```python
from build123d import *

# Parameters (mm, degrees)
F0_W     = 26
F0_H     = 15
F0_R     = 1.7
F1_DEPTH = 1.5
F2_W     = 5
F2_H     = 5
F2_R     = 1.7
F2_H_2   = 3
F3_DEPTH = 2
F4_R     = 1


with BuildPart() as f1:
    # F0 (on Top) → F1 (new body)
    with BuildSketch(Plane.XY):
        with Locations((-13, -7.5)):
            Rectangle(F0_W, F0_H)
        with Locations((-22.5, -11.9)):
            Circle(F0_R, mode=Mode.SUBTRACT)
        with Locations((-3.5, -11.9)):
            Circle(F0_R, mode=Mode.SUBTRACT)
    extrude(amount=F1_DEPTH)

    # F2 (on face) → F3 (join)
    with BuildSketch(Plane.XY.offset(1.5)):
        with Locations((-22.5, -11.9)):
            Rectangle(F2_W, F2_H)
        with Locations((-22.5, -11.9)):
            Circle(F2_R, mode=Mode.SUBTRACT)
        with Locations((-3.5, -11.9)):
            Rectangle(F2_W, F2_H)
        with Locations((-3.5, -11.9)):
            Circle(F2_R, mode=Mode.SUBTRACT)
        with Locations((-22.5, -1.5)):
            Rectangle(F2_W, F2_H_2)
        with Locations((-3.5, -1.5)):
            Rectangle(F2_W, F2_H_2)
    extrude(amount=F3_DEPTH)

    # F4
    f4_edges = [f1.edges().sort_by_distance(p)[0] for p in [
        (-26, 0, 0.75),
        (-26, -15, 0.75),
        (0, -15, 0.75),
        (0, 0, 0.75),
        (-1, -3, 2.5),
        (-6, -3, 2.5),
        (-20, -3, 2.5),
        (-25, -3, 2.5),
        (-25, -14.4, 2.5),
        (-25, -9.4, 2.5),
        (-20, -9.4, 2.5),
        (-20, -14.4, 2.5),
        (-6, -14.4, 2.5),
        (-1, -14.4, 2.5),
        (-1, -9.4, 2.5),
        (-6, -9.4, 2.5),
    ]]
    fillet(f4_edges, radius=F4_R)


solid = f1.part
```
Geometry: final body of the model. Coordinates: model frame, mm. A direction names the side the tool comes from. Round coordinates to 2 decimals unless told otherwise and drop trailing zeros. Order: outer loops, then holes, each group sorted by start corner. A loop starts at its lowest first (then second) coordinate and runs counter-clockwise, first axis right, second up. Notation, with made-up numbers: M 6,-25 L 28,-25 A29 ccw 28,-2 Z; hole C 0,-19.75 d8. An arc over 180 degrees is marked long. One line per item, written item: value.
(1) Cut plane A-A (z = 2.4). Give the number of separate pieces and of enclosed holes in the cut face, and give its area (3 significant figures).
Result sheet:
separate pieces: 4
enclosed holes: 2
area: 59.3 mm2
(2) Reachability of faces 5 (the cylindrical face through (-24.715, -9.701, 2.514)), 6 (the flat face through (-4, -9.4, 2)), 7 (the flat face through (-6, -12, 2)), 8 (the cylindrical face through (-1.285, -14.099, 2.514)), 9 (the flat face through (-13, -7, 1.5)) from +Z, -Z, +X, -X, +Y, -Y: full face, straight path, thin tool, end or side. Return the list, or none.
Result sheet:
face 5: +Z, -X
face 6: +Z, +X, -X
face 7: +Z, +Y, -Y
face 8: +Z, +X, -Y
face 9: +Z
(3) Pin query (flat end, axial travel): P1, Ø2, axis at y = -2.5, z = 3, coming from the +X side; P2, Ø1.6, axis at y = -11.5, z = 2.5, coming from the -X side; P3, Ø1.6, axis at x = -3.5, z = 3, coming from the -Y side. Return the tip coordinate at first contact, or that it passes through.
Result sheet:
P1: x = -1
P2: x = -25
P3: y = -14.4
(4) Cut plane B-B (x = -22.5). Return the cut outline in (y, z).
Result sheet:
outline: M -15,0 L -13.6,0 L -13.6,3.5 L -14.4,3.5 L -14.4,1.5 L -15,1.5 Z; M -10.2,0 L 0,0 L 0,3.5 L -3,3.5 L -3,1.5 L -9.4,1.5 L -9.4,3.5 L -10.2,3.5 Z
(5) Line query: probe 1 along Y at (x, z) = (-22.5, 2.8); probe 2 along X at (y, z) = (-11.75, 1.65); probe 3 along Y at (x, z) = (-3.5, 1.05). Output: solid intervals per line, ascending. Write a range as [from, to].
Result sheet:
probe 1: [-14.4, -13.6], [-10.2, -9.4], [-3, 0]
probe 2: [-25, -24.19], [-20.81, -20], [-6, -5.19], [-1.81, -1]
probe 3: [-15, -13.6], [-10.2, 0]
(6) Pull-direction query (X, two-part tool) for faces 1 (the flat face through (-23, -10, 3.5)), 2 (the flat face through (-6, -1, 2)), 3 (the cylindrical face through (-21.7, -13.4, 1.7)), 4 (the flat face through (-26, -8, 1)); classes: pulls with the +X half, pulls with the -X half, needs draft (parallel to the pull), parting line crosses it, or undercut.
Result sheet:
face 1: needs draft
face 2: undercut
face 3: undercut
face 4: pulls with the -X half
(7) Cut plane D-D (y = -0.75). Return the cut outline in (x, z), and give its area (3 significant figures).
Result sheet:
outline: M -25.97,0 L -0.03,0 L -0.03,1.5 L -1,1.5 L -1,3.5 L -6,3.5 L -6,1.5 L -20,1.5 L -20,3.5 L -25,3.5 L -25,1.5 L -25.97,1.5 Z
area: 58.9 mm2
(8) Cut plane C-C (y = -11.9). Return the cut outline in (x, z), and give its area (3 significant figures).
Result sheet:
outline: M -26,0 L -24.2,0 L -24.2,3.5 L -25,3.5 L -25,1.5 L -26,1.5 Z; M -20.8,0 L -5.2,0 L -5.2,3.5 L -6,3.5 L -6,1.5 L -20,1.5 L -20,3.5 L -20.8,3.5 Z; M -1.8,0 L 0,0 L 0,1.5 L -1,1.5 L -1,3.5 L -1.8,3.5 Z
area: 35.2 mm2
